The listing builds one solid part. Answer for the finished solid, in the listing's coordinates (mm). A direction names the side the tool comes from. Give positions to 0.01 mm unless a question says otherwise; leave off trailing zeros. Loops run counter-clockwise (first coordinate to the right, second up) from the corner with the lowest first, then second, coordinate; pieces in that order, holes last. Notation, with made-up numbers: M -30.5,-39.75 L -19.5,-39.75 A11 ccw -19.5,-31.75 Z; hole C 5,83.25 d11. An arc over 180 degrees is marked long. One line per item, written item: value. Start each with the question number.
Q1. Consider L1, parallel to Z at x = 32, y = 4; L2, parallel to Y at x = 1, z = -11.5; L3, parallel to X at y = 7.28, z = -19.3. Determine where each line is inside the solid, lowest interval first.
Q2. A cutting plane is placed at B-B, the plane y = 1. Determine the outline of the cut face in (x, z).
Q3. A cutting plane is placed at A-A, the plane z = -10.75. Determine the outline of the cut face in (x, y).
Q4. The mould has two halves that part along Z. Classify faces 1 (the flat face through (29.595, 9.76, -1.873)), 2 (the flat face through (17, 6, -23)), 3 (the flat face through (4.014, 3.118, -13.275)): +Z half, -Z half, draft (parallel to the pull), parting line (faces both ways), or undercut.
Q5. Flat-ended cylindrical pins translate along their axes: pin 1 (4 mm diameter, centred on x = 31, y = 7.28, fed in from -Z); pin 2 (4 mm diameter, centred on y = 4.5, z = -11, fed in from +X); pin 3 (4.5 mm diameter, centred on x = 31, y = 7.28, fed in from +Z). Find the tip coordinate at first contact, or state that the pin passes through.
Q6. A cutting plane is placed at C-C, the plane x = 19. Determine the outline of the cut face in (y, z).
Q7. A cutting plane is placed at D-D, the plane y = 6.25. State how many separate pieces and enclosed holes the cut face has, and give its area (3 significant figures).
Q8. For faces 4 (the flat face through (4.01, 9.35, -13.33)), 5 (the flat face through (23, 1, -11)), 6 (the flat face through (21, 6, -6)), 7 (the flat face through (33.85, 7, -2)), determine the directions among +Z, -Z, +X, -X, +Y, -Y from which every point of the face is accessible in a straight line to the end or side of a thin tool.
from build123d import *

# Parameters (mm, degrees)
SKETCH1_W               = 23
SKETCH1_H               = 12.5
BOSS_EXTRUDE1_DEPTH     = 35
SKETCH2_W               = 11
SKETCH2_H               = 12.5
CUT_EXTRUDE1_DEPTH      = 30
CUT_EXTRUDE2_DEPTH      = 44.706406853
CUT_EXTRUDE2_DEPTH_BACK = 44.706406853
SKETCH3_R               = 1.7
SKETCH4_R               = 2.2
CUT_EXTRUDE3_DEPTH      = 10
CUT_EXTRUDE4_DEPTH      = 2
SKETCH6_R               = 3.25
CUT_EXTRUDE5_DEPTH      = 2.5
CUT_EXTRUDE6_DEPTH      = 3.8
SKETCH8_W               = 18
SKETCH8_H               = 2
BOSS_EXTRUDE2_DEPTH     = 11
CHAMFER2_SIZE           = 1.5


with BuildPart() as part:
    # Sketch1 → Boss-Extrude1 (new body)
    with BuildSketch(Plane(origin=(0, 0, 0), x_dir=(0, 0, -1), z_dir=(1, 0, 0))):
        with Locations((11.5, 6.25)):
            Rectangle(SKETCH1_W, SKETCH1_H)
    extrude(amount=BOSS_EXTRUDE1_DEPTH)

    # Sketch2 → Cut-Extrude1 (cut)
    with BuildSketch(Plane(origin=(35, 0, 0), x_dir=(0, 0, -1), z_dir=(1, 0, 0))):
        with Locations((11.5, 6.25)):
            Rectangle(SKETCH2_W, SKETCH2_H)
    extrude(amount=-CUT_EXTRUDE1_DEPTH, mode=Mode.SUBTRACT)

    # Sketch3 → Cut-Extrude2 (cut, two sides: drawn at the far end of the back side and taken through both)
    with BuildSketch(Plane(origin=(0, 0, -23), x_dir=(-1, 0, 0), z_dir=(0, 0, -1)).offset(-CUT_EXTRUDE2_DEPTH_BACK)):
        with Locations(Location((-31, 7.28, 0), (0, 0, 90))):
            Circle(SKETCH3_R)
    extrude(amount=CUT_EXTRUDE2_DEPTH + CUT_EXTRUDE2_DEPTH_BACK, mode=Mode.SUBTRACT)

    # Sketch4 → Cut-Extrude3 (cut)
    with BuildSketch(Plane.ZY):
        with Locations((-11.5, 6.25)):
            Circle(SKETCH4_R)
    extrude(amount=-CUT_EXTRUDE3_DEPTH, mode=Mode.SUBTRACT)

    # Sketch5 → Cut-Extrude4 (cut)
    with BuildSketch(Plane(origin=(5, 0, 0), x_dir=(0, 0, -1), z_dir=(1, 0, 0))):
        Polygon((7.9, 8.328460969), (7.9, 4.171539031), (11.5, 2.093078062), (15.1, 4.171539031), (15.1, 8.328460969), (11.5, 10.406921938), align=None)
    extrude(amount=-CUT_EXTRUDE4_DEPTH, mode=Mode.SUBTRACT)

    # Sketch6 → Cut-Extrude5 (cut)
    with BuildSketch(Plane(origin=(0, 0, -23), x_dir=(-1, 0, 0), z_dir=(0, 0, -1))):
        with Locations((-31, 7.28)):
            Circle(SKETCH6_R)
    extrude(amount=-CUT_EXTRUDE5_DEPTH, mode=Mode.SUBTRACT)

    # Sketch7 → Cut-Extrude6 (cut)
    with BuildSketch(Plane.XY):
        Polygon((28.15, 8.925448267), (28.15, 5.634551733), (31, 3.989103466), (33.85, 5.634551733), (33.85, 8.925448267), (31, 10.570896534), align=None)
    extrude(amount=-CUT_EXTRUDE6_DEPTH, mode=Mode.SUBTRACT)

    # Sketch8 → Boss-Extrude2 (add)
    with BuildSketch(Plane(origin=(0, 0, -6), x_dir=(-1, 0, 0), z_dir=(0, 0, -1))):
        with Locations((-14, 1)):
            Rectangle(SKETCH8_W, SKETCH8_H)
    extrude(amount=BOSS_EXTRUDE2_DEPTH)

    # Chamfer2
    chamfer2_edges = [part.edges().sort_by_distance(p)[0] for p in [
        (5, 7.25, -6),
        (5, 7.25, -17),
    ]]
    chamfer(chamfer2_edges, length=CHAMFER2_SIZE)


solid = part.part
Answer block:
1. L1: -23 to -17, -6 to 0
1. L2: 0 to 4.05, 8.45 to 12.5
1. L3: 0 to 29.3, 32.7 to 35
2. outline: M 0,-23 L 35,-23 L 35,-17 L 23,-17 L 23,-6 L 35,-6 L 35,0 L 0,0 Z
3. outline: M 0,0 L 23,0 L 23,2 L 5,2 L 5,2.53 L 3,2.53 L 3,4.18 L 0,4.18 Z; M 0,8.32 L 3,8.32 L 3,9.97 L 5,9.97 L 5,12.5 L 0,12.5 Z
4. face 1: draft
4. face 2: -Z half
4. face 3: undercut
5. pin 1: z = -20.5
5. pin 2: x = 5
5. pin 3: z = -3.8
6. outline: M 0,-23 L 12.5,-23 L 12.5,-17 L 2,-17 L 2,-6 L 12.5,-6 L 12.5,0 L 0,0 Z
7. separate pieces: 4
7. enclosed holes: 0
7. area: 397 mm^2
8. face 4: +X
8. face 5: +X, +Y, -Y
8. face 6: +X, +Y
8. face 7: +Z
